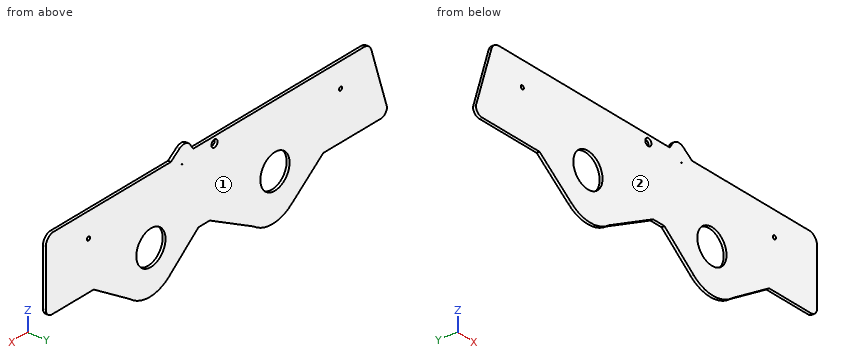
```python
from build123d import *

# Parameters (mm, degrees)
SKETCH1_R                = 4.6
BOSS_EXTRUDE1_DEPTH      = 3.175
SKETCH2_W                = 597.466303312
SKETCH2_H                = 60.972543052
CUT_EXTRUDE1_DEPTH       = 70
FILLET1_R                = 10
FILLET2_R                = 10
SKETCH3_R                = 3.990837639
CUT_EXTRUDE2_DEPTH       = 10
SKETCH4_R                = 2
CUT_EXTRUDE3_DEPTH       = 470.13785887
SKETCH5_R                = 2
CUT_EXTRUDE4_DEPTH       = 10
SKETCH6_R                = 40
BOSS_EXTRUDE2_DEPTH      = 3.175
BOSS_EXTRUDE3_DEPTH      = 3.175
SKETCH9_R                = 40
BOSS_EXTRUDE4_DEPTH      = 3.175
BOSS_EXTRUDE6_DEPTH      = 3.175
SKETCH13_R               = 19
CUT_EXTRUDE5_DEPTH       = 10
SKETCH14_R               = 19
CUT_EXTRUDE6_DEPTH       = 10
BOSS_EXTRUDE7_DEPTH      = 10
BOSS_EXTRUDE7_DEPTH_BACK = 3.175
SKETCH16_W               = 39.380598922
SKETCH16_H               = 33.904845405
CUT_EXTRUDE7_DEPTH       = 10


with BuildPart() as part:
    # Sketch1 → Boss-Extrude1 (new body)
    with BuildSketch(Plane(origin=(0, 0, 0), x_dir=(1, 0, 0), z_dir=(0, 1, 0))):
        with BuildLine():
            ThreePointArc((8, 150), (2.343145751, 147.656854249), (0, 142))
            Line((0, 142), (42, 8))
            ThreePointArc((42, 8), (44.343145751, 2.343145751), (50, 0))
            Line((50, 0), (436.5, 0))
            ThreePointArc((436.5, 0), (442.156854249, 2.343145751), (444.5, 8))
            Line((444.5, 8), (444.5, 142))
            ThreePointArc((444.5, 142), (442.156854249, 147.656854249), (436.5, 150))
            Line((436.5, 150), (172.868406334, 150))
            ThreePointArc((172.868406334, 150), (172.5, 146.64039861), (172.131593666, 150))
            Line((172.131593666, 150), (8, 150))
        make_face()
        with Locations(Location((265.281257274, 74.563866981, 0), (0, 0, 270))):
            Circle(SKETCH1_R, mode=Mode.SUBTRACT)
    extrude(amount=BOSS_EXTRUDE1_DEPTH)

    # Sketch2 → Cut-Extrude1 (cut)
    with BuildSketch(Plane.XY):
        with Locations((220.1785332, 7.544358636)):
            Rectangle(SKETCH2_W, SKETCH2_H)
    extrude(amount=-CUT_EXTRUDE1_DEPTH, mode=Mode.SUBTRACT)

    # Fillet1
    fillet1_edges = [part.edges().sort_by_distance(p)[0] for p in [
        (22.567164179, 1.5875, -70),
    ]]
    fillet(fillet1_edges, radius=FILLET1_R)

    # Fillet2
    fillet2_edges = [part.edges().sort_by_distance(p)[0] for p in [
        (444.5, 1.5875, -70),
    ]]
    fillet(fillet2_edges, radius=FILLET2_R)

    # Sketch3 → Cut-Extrude2 (cut)
    with BuildSketch(Plane(origin=(0, 3.175, 0), x_dir=(1, 0, 0), z_dir=(0, 1, 0))):
        with Locations(Location((224.75, 77.255, 0), (0, 0, 270))):
            Circle(SKETCH3_R)
    extrude(amount=-CUT_EXTRUDE2_DEPTH, mode=Mode.SUBTRACT)

    # Sketch4 → Cut-Extrude3 (cut, through all)
    with BuildSketch(Plane(origin=(0, 3.175, 0), x_dir=(1, 0, 0), z_dir=(0, 1, 0))):
        with Locations(Location((60.5, 97, 0), (0, 0, 270))):
            Circle(SKETCH4_R)
    extrude(amount=-CUT_EXTRUDE3_DEPTH, mode=Mode.SUBTRACT)

    # Sketch5 → Cut-Extrude4 (cut)
    with BuildSketch(Plane(origin=(0, 3.175, 0), x_dir=(1, 0, 0), z_dir=(0, 1, 0))):
        with Locations(Location((389, 97, 0), (0, 0, 270))):
            Circle(SKETCH5_R)
    extrude(amount=-CUT_EXTRUDE4_DEPTH, mode=Mode.SUBTRACT)

    # Sketch6 → Boss-Extrude2 (add)
    with BuildSketch(Plane(origin=(0, 0, 0), x_dir=(1, 0, 0), z_dir=(0, 1, 0))):
        with Locations((149, 150.04039861)):
            Circle(SKETCH6_R)
    extrude(amount=BOSS_EXTRUDE2_DEPTH)

    # Sketch7 → Boss-Extrude3 (add)
    with BuildSketch(Plane(origin=(0, 0, 0), x_dir=(1, 0, 0), z_dir=(0, 1, 0))):
        Polygon((124.164543783, 181.396420591), (82.702881078, 149.750534228), (231.468946681, 149.750534228), (173.835456217, 181.396420591), align=None)
    extrude(amount=BOSS_EXTRUDE3_DEPTH)

    # Sketch9 → Boss-Extrude4 (add)
    with BuildSketch(Plane(origin=(0, 0, 0), x_dir=(1, 0, 0), z_dir=(0, 1, 0))):
        with BuildLine():
            ThreePointArc((269, 150), (272.870833001, 167.166341835), (283.734164599, 181.010281545))
            Line((283.734164599, 181.010281545), (245.673378314, 150))
            Line((245.673378314, 150), (269, 150))
        make_face()
        with Locations((309, 150)):
            Circle(SKETCH9_R)
    extrude(amount=BOSS_EXTRUDE4_DEPTH)

    # Sketch12 → Boss-Extrude6 (add)
    with BuildSketch(Plane(origin=(0, 0, 0), x_dir=(1, 0, 0), z_dir=(0, 1, 0))):
        Polygon((326.166341835, 186.129166999), (382.106475607, 150), (340.398839744, 150), align=None)
    extrude(amount=BOSS_EXTRUDE6_DEPTH)

    # Sketch13 → Cut-Extrude5 (cut)
    with BuildSketch(Plane(origin=(0, 3.175, 0), x_dir=(1, 0, 0), z_dir=(0, 1, 0))):
        with Locations(Location((146, 139.84039861, 0), (0, 0, 270))):
            Circle(SKETCH13_R)
    extrude(amount=-CUT_EXTRUDE5_DEPTH, mode=Mode.SUBTRACT)

    # Sketch14 → Cut-Extrude6 (cut)
    with BuildSketch(Plane(origin=(0, 3.175, 0), x_dir=(1, 0, 0), z_dir=(0, 1, 0))):
        with Locations(Location((307.606475607, 142.298064477, 0), (0, 0, 270))):
            Circle(SKETCH14_R)
    extrude(amount=-CUT_EXTRUDE6_DEPTH, mode=Mode.SUBTRACT)

    # Sketch15 → Boss-Extrude7 (add, two sides: drawn at the far end of the back side and taken through both)
    with BuildSketch(Plane(origin=(0, 3.175, 0), x_dir=(1, 0, 0), z_dir=(0, 1, 0)).offset(-BOSS_EXTRUDE7_DEPTH_BACK)):
        with BuildLine():
            Line((270.323640372, 61.870718801), (281.671389991, 70))
            Line((281.671389991, 70), (265.856685963, 70))
            ThreePointArc((265.856685963, 70), (269.551101507, 72.852601302), (268.849345077, 77.467097842))
            Line((268.849345077, 77.467097842), (266.045546336, 79.099929396))
            ThreePointArc((266.045546336, 79.099929396), (260.730312777, 75.233870106), (264.705828584, 70))
            Line((264.705828584, 70), (252.589726142, 70))
            Line((252.589726142, 70), (257.164027826, 63.204154779))
            ThreePointArc((257.164027826, 63.204154779), (263.491883069, 60.050944756), (270.323640372, 61.870718801))
        make_face()
    extrude(amount=BOSS_EXTRUDE7_DEPTH + BOSS_EXTRUDE7_DEPTH_BACK)

    # Sketch16 → Cut-Extrude7 (cut)
    with BuildSketch(Plane(origin=(0, 13.175, 0), x_dir=(1, 0, 0), z_dir=(0, 1, 0))):
        with Locations((267.135263248, 68.050551455)):
            Rectangle(SKETCH16_W, SKETCH16_H)
    extrude(amount=-CUT_EXTRUDE7_DEPTH, mode=Mode.SUBTRACT)


solid = part.part
```
The listing builds one solid part. Answer for the finished solid, in the listing's coordinates (mm). Face numbers are marked on the shaded views. Coordinates: 2 decimals unless noted, no trailing zeros. Loops run counter-clockwise (first coordinate to the right, second up) from the corner with the lowest first, then second, coordinate; pieces in that order, holes last. Notation, with made-up numbers: (42, 29) - (83, 29) arc R29 ccw to (83, 50) - close; hole circle Ø10 at (30.25, -5). An arc over 180 degrees is marked (long way). Use a Markdown table: item, result. Add a question column.
1) The mould has two halves that part along Y. Classify the marked faces 1 and 2: released by +Y, released by -Y, zero draft, split by the parting line, or undercut.
2) The part is cut by section D-D, the plane x = 146. Give the vertices of the cut face in (y, z) (3 decimals), and give its area (3 significant figures).
3) Find the intervals of material crossed by line 1 (X direction, y = 0.3, z = -152); line 2 (Z direction, x = 389, y = 1.5); line 3 (X direction, y = 1.65, z = -144), in increasing order.
4) The part is cut by section B-B, the plane y = 0.8. Give the vertices of the cut face in (x, z) (3 decimals).
5) The part is cut by section C-C, the plane z = -128. Give the vertices of the cut face in (x, y) (1 decimal), and give its area (3 significant figures).
6) The part is cut by section A-A, the plane x = 224.75. Give the vertices of the cut face in (y, z) (3 decimals), and give its area (3 significant figures).
7) Given pin 1 (1.5 mm diameter, centred on y = 1, z = -143, fed in from -X); pin 2 (1 mm diameter, centred on x = 407, y = 1.5, fed in from -Z); pin 3 (4.5 mm diameter, centred on x = 60.5, z = -97, fed in from -Y); pin 4 (1.6 mm diameter, centred on x = 151.5, y = 2, fed in from +Z), each flat-ended and moving along its own axis, determine where each tip first touches the part or whether it passes through.
Here are the results:
| question | item | result |
|---|---|---|
| 1 | face 1 | released by +Y |
| 1 | face 2 | released by -Y |
| 2 | outline | (0, -189.928) - (3.175, -189.928) - (3.175, -158.84) - (0, -158.84) - close; (0, -120.84) - (3.175, -120.84) - (3.175, -70) - (0, -70) - close |
| 2 | area | 260 mm^2 |
| 3 | line 1 | x = 85.65 to 131.4, 160.6 to 227.37, 248.13 to 291.27, 323.94 to 379.01 |
| 3 | line 2 | z = -150 to -99, -95 to -70 |
| 3 | line 3 | x = 0.25 to 127.46, 164.54 to 288.68, 326.53 to 444.25 |
| 4 | outline | (0, -142) arc R8 ccw to (8, -150) - (83.03, -150) - (124.165, -181.396) arc R40 ccw to (173.835, -181.396) - (231.015, -150) - (245.673, -150) - (283.734, -181.01) arc R40 ccw to (334.871, -180.507) - (382.106, -150) - (436.5, -150) arc R8 ccw to (444.5, -142) - (444.5, -80) arc R10 ccw to (434.5, -70) - (281.671, -70) - (270.324, -61.871) arc R10 ccw to (257.164, -63.204) - (252.59, -70) - (29.913, -70) arc R10 ccw to (20.37, -77.009) - close; hole circle Ø4 at (60.5, -97); hole circle Ø38 at (146, -139.84); hole circle Ø7.982 at (224.75, -77.255); hole (266.046, -79.1) arc R4.6 ccw to (268.849, -77.467) - close; hole circle Ø38 at (307.606, -142.298); hole circle Ø4 at (389, -97) |
| 5 | outline | (4.4, 0) - (131.1, 0) - (131.1, 3.2) - (4.4, 3.2) - close; (160.9, 0) - (295.1, 0) - (295.1, 3.2) - (160.9, 3.2) - close; (320.1, 0) - (444.5, 0) - (444.5, 3.2) - (320.1, 3.2) - close |
| 5 | area | 1,220 mm^2 |
| 6 | outline | (0, -153.44) - (3.175, -153.44) - (3.175, -81.246) - (0, -81.246) - close; (0, -73.264) - (3.175, -73.264) - (3.175, -70) - (0, -70) - close |
| 6 | area | 240 mm^2 |
| 7 | pin 1 | stops at x = 0 |
| 7 | pin 2 | stops at z = -150 |
| 7 | pin 3 | stops at y = 0 |
| 7 | pin 4 | stops at z = -70 |
